CAD build for the part. Positions are in the model's coordinates, mm. A direction names the side the tool comes from. Coordinates: 2 decimals unless noted, no trailing zeros. Loops run counter-clockwise (first coordinate to the right, second up) from the corner with the lowest first, then second, coordinate; pieces in that order, holes last. Notation, with made-up numbers: (83, -13) -> (88, -13) arc R26 ccw to (88, 10) -> close; hole circle Ø6 at (15.5, -36.5). An arc over 180 degrees is marked (long way). Answer as CSV lines item,"result". Start each with the question number.
```python
from build123d import *

# Parameters (mm, degrees)
F1_DEPTH = 50
F3_D     = 3.5
F4_R     = 2.4
F4_R_2   = 1.75
F5_DEPTH = 2


with BuildPart() as f1:
    # F0 (on Front) → F1 (new body, symmetric)
    with BuildSketch(Plane.XZ):
        Polygon((-9.9684563031, 8.1134089709), (-9.9684563031, -6.8865910291), (-4.9684563031, -6.8865910291), (-4.9684563031, 3.1134089709), (20.0315436969, 3.1134089709), (20.0315436969, 8.1134089709), align=None)
    extrude(amount=F1_DEPTH, both=True)

    # F3 (through all)
    with Locations(Plane.YZ.offset(-4.9684563031)):
        with Locations((-25, -1.8865910291), (25, -1.8865910291)):
            Hole(F3_D / 2)

    # F4 (on face) → F5 (cut)
    with BuildSketch(Plane.YZ.offset(-4.9684563031)):
        with Locations((-25, -1.8865910291)):
            Circle(F4_R)
        with Locations((-25, -1.8865910291)):
            Circle(F4_R_2, mode=Mode.SUBTRACT)
        with Locations((25, -1.8865910291)):
            Circle(F4_R)
        with Locations((25, -1.8865910291)):
            Circle(F4_R_2, mode=Mode.SUBTRACT)
    extrude(amount=-F5_DEPTH, mode=Mode.SUBTRACT)


solid = f1.part
```
Q1. Saw through at B-B (y = 42). List the corners of the cut face in (x, z), and give its area (3 significant figures).
Q2. Pin check, flat tips, straight feed: pin 1 Ø4 at (y, z) = (-25, -1.89) entering from +X; pin 2 Ø7.5 at (x, y) = (2.5, 13.5) entering from -Z; pin 3 Ø5.5 at (y, z) = (-25.5, -2.5) entering from +X. Stop position of each tip, or through.
Q3. Probe probe 1 along Z at (x, y) = (-8, 25); probe 2 along Z at (x, y) = (-5.45, -25); probe 3 along Y at (x, z) = (-5, 0). List the from-to ranges inside material, lowest first. Write a range as from..to.
Q4. Saw through at C-C (x = 0). List the corners of the cut face in (y, z), and give its area (3 significant figures).
Q5. Two-plate mould, pull along Y, no slides. Class faces 4 (the flat face through (-8, -1, -6.887)), 5 (the flat face through (1, 50, 4)), 6 (the flat face through (-6.968, 25, -4)), 7 (the cylindrical face through (-8.49, -23.25, -1.81)): pulls with the +Y half, pulls with the -Y half, needs draft (parallel to the pull), parting line crosses it, or undercut.
Q6. Which spindle directions (+Z, -Z, +X, -X, +Y, -Y) get a long thin tool onto all of the face, cutting with end or side? Do faces 1 (the flat face through (7, -1, 3.113)), 2 (the flat face through (5, -1, 8.113)), 3 (the cylindrical face through (-6, -22.7, -1.2)). Say none if no direction does.
Q7. Saw through at A-A (y = -25). List the corners of the cut face in (x, z), and give its area (3 significant figures).
Ans:
1,outline,"(-9.97, -6.89) -> (-4.97, -6.89) -> (-4.97, 3.11) -> (20.03, 3.11) -> (20.03, 8.11) -> (-9.97, 8.11) -> close"
1,area,"200 mm²"
2,pin 1,"stops at x = -6.97"
2,pin 2,"stops at z = 3.11"
2,pin 3,"stops at x = -4.97"
3,probe 1,"z = -6.89..-3.64, -0.14..8.11"
3,probe 2,"z = -6.89..-4.29, 0.51..8.11"
3,probe 3,"y = -50..-26.48, -23.52..23.52, 26.48..50"
4,outline,"(-50, 3.11) -> (50, 3.11) -> (50, 8.11) -> (-50, 8.11) -> close"
4,area,"500 mm²"
5,face 4,"needs draft"
5,face 5,"pulls with the +Y half"
5,face 6,"undercut"
5,face 7,"undercut"
6,face 1,"-Z, +X, +Y, -Y"
6,face 2,"+Z, +X, -X, +Y, -Y"
6,face 3,"+X"
7,outline,"(-9.97, -6.89) -> (-4.97, -6.89) -> (-4.97, -4.29) -> (-6.97, -4.29) -> (-6.97, -3.64) -> (-9.97, -3.64) -> close; (-9.97, -0.14) -> (-6.97, -0.14) -> (-6.97, 0.51) -> (-4.97, 0.51) -> (-4.97, 3.11) -> (20.03, 3.11) -> (20.03, 8.11) -> (-9.97, 8.11) -> close"
7,area,"180 mm²"
